from build123d import *
from OCP.BRepFilletAPI import BRepFilletAPI_MakeChamfer

# Parameters (mm, degrees)
BOSS_EXTRUDE1_DEPTH = 10
CHAMFER1_SIZE       = 10
CHAMFER1_SIZE_2     = 2.308681911


with BuildPart() as part:
    # Sketch1 → Boss-Extrude1 (new body)
    with BuildSketch(Plane(origin=(0, 0, 0), x_dir=(1, 0, 0), z_dir=(0, 1, 0))):
        with BuildLine():
            Line((-306, 0), (306, 0))
            Line((306, 0), (22.078307516, -504.188415778))
            ThreePointArc((22.078307516, -504.188415778), (0, -498.4), (-22.078307516, -504.188415778))
            Line((-22.078307516, -504.188415778), (-306, 0))
        make_face()
    extrude(amount=BOSS_EXTRUDE1_DEPTH)

    # Chamfer1
    chamfer1_edges_1 = [part.edges().sort_by_distance(p)[0] for p in [
        (-164.039153758, 0, 252.094207889),
    ]]
    chamfer1_side_1 = [part.faces().sort_by_distance(p)[0] for p in [
        (-164.039153758, 0.046173638, 252.094207889),
    ]]
    chamfer1_edges_2 = [part.edges().sort_by_distance(p)[0] for p in [
        (0, 0, 0),
    ]]
    chamfer1_side_2 = [part.faces().sort_by_distance(p)[0] for p in [
        (0, 0.046173638, 0),
    ]]
    chamfer1_edges_3 = [part.edges().sort_by_distance(p)[0] for p in [
        (164.039153758, 0, 252.094207889),
    ]]
    chamfer1_side_3 = [part.faces().sort_by_distance(p)[0] for p in [
        (164.039153758, 0.046173638, 252.094207889),
    ]]
    chamfer1 = BRepFilletAPI_MakeChamfer(part.part.solid().wrapped)
    for e in chamfer1_edges_1:
        chamfer1.Add(CHAMFER1_SIZE - 0.0001, CHAMFER1_SIZE_2 - 0.0001, e.wrapped, chamfer1_side_1[0].wrapped)
    for e in chamfer1_edges_2:
        chamfer1.Add(CHAMFER1_SIZE - 0.0001, CHAMFER1_SIZE_2 - 0.0001, e.wrapped, chamfer1_side_2[0].wrapped)
    for e in chamfer1_edges_3:
        chamfer1.Add(CHAMFER1_SIZE - 0.0001, CHAMFER1_SIZE_2 - 0.0001, e.wrapped, chamfer1_side_3[0].wrapped)
    add(Compound.cast(chamfer1.Shape()), mode=Mode.REPLACE)  # a hair under: the kernel refuses the full size


solid = part.part
Geometry check sheet. Reference: the model listing, model coordinates, mm. Round coordinates to 2 decimals unless told otherwise and drop trailing zeros. Order: outer loops, then holes, each group sorted by start corner. A loop starts at its lowest first (then second) coordinate and runs counter-clockwise, first axis right, second up. Notation, with made-up numbers: (-20, 61) - (-1, 61) arc R19 cw to (-1, 83) - close; hole circle Ø10 at (57, 71.25). An arc over 180 degrees is marked (long way). One line per question, with ' | ' between items. Start each with the question number.
(1) Sectioned sample at C-C on y = 2. Record the cut outline in (x, z).
(2) Thickness scan on L1, parallel to Z at x = 213, y = 5; L2, parallel to X at y = 9.75, z = 206.5; L3, parallel to Z at x = 205, y = 2. Record the ranges inside material, lowest first. Write a range as [from, to].
(3) Depth check by flat-ended pin: pin 1 Ø6 at (x, y) = (116.5, 8) entering from -Z; pin 2 Ø1.5 at (x, y) = (124, 2.5) entering from +Z; pin 3 Ø5 at (y, z) = (3.5, 439.5) entering from +X. Enter the tip coordinate at first touch or a pass-through.
Conclusion:
1) outline: (-302.84, 1.85) - (302.84, 1.85) - (20.45, 503.32) arc R45 cw to (-20.45, 503.32) - close
2) L1: z = [1.15, 162.8] | L2: x = [-189.65, 189.65] | L3: z = [1.85, 175.59]
3) pin 1: stops at z = 0 | pin 2: stops at z = 321.04 | pin 3: stops at x = 58.34
